Here's how the part is built. I have some questions about the finished solid (model axes, mm). Face numbers are marked on the shaded views. A direction names the side the tool comes from. Round coordinates to 2 decimals unless told otherwise and drop trailing zeros. Write each loop counter-clockwise with the first axis right and the second up, starting at its lowest first coordinate (ties: lowest second). Pieces come first, ordered by that corner, then holes. Notation, with made-up numbers: (78.25, 41.5) -> (125.25, 41.5) arc R25 ccw to (125.25, 53.5) -> close; hole circle Ø11 at (23, 72). An arc over 180 degrees is marked (long way). Answer in a Markdown table with one row per item.
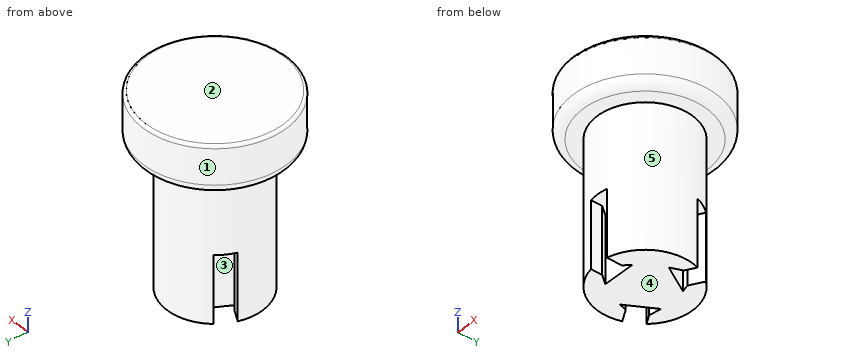
from build123d import *

# Parameters (mm, degrees)
F0_R     = 9.525
F1_DEPTH = 6.35
F2_R     = 6.35
F3_DEPTH = 19.05
F5_DEPTH = 8.89
F6_R     = 1.27
F7_R     = 0.381


with BuildPart() as f1:
    # F0 (on Top) → F1 (new body)
    with BuildSketch(Plane.XY):
        Circle(F0_R)
    extrude(amount=F1_DEPTH)

    # F2 (on face) → F3 (join)
    with BuildSketch(Plane(origin=(0, 0, 0), x_dir=(1, 0, 0), z_dir=(0, 0, -1))):
        Circle(F2_R)
    extrude(amount=F3_DEPTH)

    # F4 (on face) → F5 (cut)
    with BuildSketch(Plane(origin=(0, 0, -19.05), x_dir=(1, 0, 0), z_dir=(0, 0, -1))):
        with BuildLine():
            ThreePointArc((1.27, 6.2217039467), (0.6382319087, 6.3178445716), (0, 6.35))
            ThreePointArc((0, 6.35), (-0.6382319087, 6.3178445716), (-1.27, 6.2217039467))
            Line((-1.27, 6.2217039467), (-1.27, 4.699))
            Line((-1.27, 4.699), (-2.286, 3.429))
            Line((-2.286, 3.429), (1.27, 3.429))
            Line((1.27, 3.429), (2.032, 3.429))
            Line((2.032, 3.429), (1.27, 4.191))
            Line((1.27, 4.191), (1.27, 6.2217039467))
        make_face()
        with BuildLine():
            Line((-4.2645124673, -0.9956477372), (-6.0231536726, -2.0109997105))
            ThreePointArc((-6.0231536726, -2.0109997105), (-5.7905298505, -2.6061972393), (-5.499261314, -3.175))
            ThreePointArc((-5.499261314, -3.175), (-5.1522979418, -3.7116473323), (-4.7531536726, -4.2107042361))
            Line((-4.7531536726, -4.2107042361), (-3.4344533724, -3.4493522628))
            Line((-3.4344533724, -3.4493522628), (-1.8266011096, -3.6942340731))
            Line((-1.8266011096, -3.6942340731), (-3.9856011096, 0.0452636205))
            Line((-3.9856011096, 0.0452636205), (-4.2645124673, -0.9956477372))
        make_face()
        with BuildLine():
            ThreePointArc((5.499261314, -3.175), (5.7905298505, -2.6061972393), (6.0231536726, -2.0109997105))
            Line((6.0231536726, -2.0109997105), (4.7044533724, -1.2496477372))
            Line((4.7044533724, -1.2496477372), (4.1126011096, 0.2652340731))
            Line((4.1126011096, 0.2652340731), (1.9536011096, -3.4742636205))
            Line((1.9536011096, -3.4742636205), (2.9945124673, -3.1953522628))
            Line((2.9945124673, -3.1953522628), (4.7531536726, -4.2107042361))
            ThreePointArc((4.7531536726, -4.2107042361), (5.1522979418, -3.7116473323), (5.499261314, -3.175))
        make_face()
    extrude(amount=-F5_DEPTH, mode=Mode.SUBTRACT)

    # F6
    f6_edges = [f1.edges().sort_by_distance(p)[0] for p in [
        (-9.525, 0, 0),
    ]]
    fillet(f6_edges, radius=F6_R)

    # F7
    f7_edges = [f1.edges().sort_by_distance(p)[0] for p in [
        (-9.525, 0, 6.35),
    ]]
    fillet(f7_edges, radius=F7_R)


solid = f1.part
1) We'd pull the mould along X, two halves only. Please class the marked faces 1, 2 and 3: +X half, -X half, draft (parallel to the pull), parting line (faces both ways), or undercut.
Response:
| item | result |
|---|---|
| face 1 | parting line |
| face 2 | draft |
| face 3 | undercut |
2) Which directions (+Z, -Z, +X, -X, +Y, -Y) give clear straight access to the entire face, cutting with the end or side of a thin tool? Please do the marked faces 4 and 5.
Response:
| item | result |
|---|---|
| face 4 | -Z, +X, -X, +Y, -Y |
| face 5 | -Z |
3) I want a section at B-B, the plane z = -17.5. List the corners of the cut face in (x, y) for me.
Response:
| item | result |
|---|---|
| outline | (-6.02, 2.01) arc R6.35 ccw to (-1.27, -6.22) -> (-1.27, -4.7) -> (-2.29, -3.43) -> (2.03, -3.43) -> (1.27, -4.19) -> (1.27, -6.22) arc R6.35 ccw to (6.02, 2.01) -> (4.7, 1.25) -> (4.11, -0.27) -> (1.95, 3.47) -> (2.99, 3.2) -> (4.75, 4.21) arc R6.35 ccw to (-4.75, 4.21) -> (-3.43, 3.45) -> (-1.83, 3.69) -> (-3.99, -0.05) -> (-4.26, 1) -> close |
4) I want a section at C-C, the plane z = -2.25. List the corners of the cut face in (x, y) for me.
Response:
| item | result |
|---|---|
| outline | circle Ø12.7 at (0, 0) |
5) For pin 1 (0.8 mm diameter, centred on y = -5.5, z = -15.5, fed in from +X); pin 2 (1.2 mm diameter, centred on x = 4, y = 2, fed in from -Z); pin 3 (6 mm diameter, centred on y = -7.5, z = 3, fed in from -X) (3 decimals), each with a flat end and sliding along its axis, tell me the tip position at first contact or that it passes through.
Response:
| item | result |
|---|---|
| pin 1 | stops at x = 3.78 |
| pin 2 | stops at z = -10.16 |
| pin 3 | stops at x = -8.395 |
6) I want a section at A-A, the plane x = 0. List the corners of the cut face in (y, z) for me (3 decimals), and give its area (3 significant figures).
Response:
| item | result |
|---|---|
| outline | (-9.525, 1.27) arc R1.27 ccw to (-8.255, 0) -> (-6.35, 0) -> (-6.35, -10.16) -> (-3.429, -10.16) -> (-3.429, -19.05) -> (6.35, -19.05) -> (6.35, 0) -> (8.255, 0) arc R1.27 ccw to (9.525, 1.27) -> (9.525, 5.969) arc R0.381 ccw to (9.144, 6.35) -> (-9.144, 6.35) arc R0.381 ccw to (-9.525, 5.969) -> close |
| area | 336 mm^2 |
7) I need wall thicknesses on line 1 (Y direction, x = -0.25, z = -12); line 2 (X direction, y = 0.75, z = -13.5); line 3 (Z direction, x = 1.75, y = 6.75). Which ranges of each line are inside material? Lowest first, please. Write a range as [from, to].
Response:
| item | result |
|---|---|
| line 1 | y = [-3.43, 6.35] |
| line 2 | x = [-6.31, -4.2], [-3.53, 3.53], [4.51, 6.31] |
| line 3 | z = [0, 6.35] |
